```python
from build123d import *

# Parameters (mm, degrees)
SKETCH1_W                 = 105
SKETCH1_H                 = 65
BOSS_EXTRUDE1_DEPTH       = 40
FILLET1_R                 = 5
CUT_EXTRUDE1_DEPTH        = 38
SKETCH4_R                 = 2.5
SKETCH4_R_2               = 1
BOSS_EXTRUDE2_DEPTH       = 30
MIRROR2_COPY_1_SKETCH_R   = 2.5
MIRROR2_COPY_1_SKETCH_R_2 = 1
MIRROR2_COPY_1_DEPTH      = 30
CUT_EXTRUDE2_REACH        = 67
SKETCH7_R                 = 1.5
CUT_EXTRUDE3_REACH        = 4
SKETCH9_R                 = 2
CUT_EXTRUDE4_REACH        = 67
SKETCH12_R                = 3
FILLET2_R                 = 1
CUT_EXTRUDE5_REACH        = 67
SKETCH13_R                = 1.75


with BuildPart() as part:
    # Sketch1 → Boss-Extrude1 (new body)
    with BuildSketch(Plane(origin=(0, 0, 0), x_dir=(1, 0, 0), z_dir=(0, 1, 0))):
        with Locations((52.5, 32.5)):
            Rectangle(SKETCH1_W, SKETCH1_H)
    extrude(amount=BOSS_EXTRUDE1_DEPTH)

    # Fillet1
    fillet1_edges = [part.edges().sort_by_distance(p)[0] for p in [
        (0, 20, 0),
        (0, 20, -65),
        (105, 20, -65),
        (105, 20, 0),
    ]]
    fillet(fillet1_edges, radius=FILLET1_R)

    # Sketch3 → Cut-Extrude1 (cut)
    with BuildSketch(Plane(origin=(0, 40, 0), x_dir=(1, 0, 0), z_dir=(0, 1, 0))):
        with BuildLine():
            Line((100, 63), (5, 63))
            ThreePointArc((5, 63), (2.878679656, 62.121320344), (2, 60))
            Line((2, 60), (2, 5))
            ThreePointArc((2, 5), (2.878679656, 2.878679656), (5, 2))
            Line((5, 2), (100, 2))
            ThreePointArc((100, 2), (102.121320344, 2.878679656), (103, 5))
            Line((103, 5), (103, 60))
            ThreePointArc((103, 60), (102.121320344, 62.121320344), (100, 63))
        make_face()
    extrude(amount=-CUT_EXTRUDE1_DEPTH, mode=Mode.SUBTRACT)

    # Sketch4 → Boss-Extrude2 (add)
    with BuildSketch(Plane(origin=(0, 2, 0), x_dir=(1, 0, 0), z_dir=(0, 1, 0))):
        with Locations((99, 6)):
            Circle(SKETCH4_R)
        with Locations((99, 6)):
            Circle(SKETCH4_R_2, mode=Mode.SUBTRACT)
    boss_extrude2 = extrude(amount=BOSS_EXTRUDE2_DEPTH)

    # Mirror1: Boss-Extrude2 across plane
    add(boss_extrude2.mirror(Plane(origin=(0, 0, -32.5), x_dir=(1, 0, 0), z_dir=(0, 0, -1))))

    # Mirror2: Boss-Extrude2 across plane
    add(boss_extrude2.mirror(Plane.ZY.offset(-52.5)))

    # Mirror2 copy 1 sketch → Mirror2 copy 1 (add)
    with BuildSketch(Plane(origin=(105, 2, -65), x_dir=(-1, 0, 0), z_dir=(0, 1, 0))):
        with Locations((99, 6)):
            Circle(MIRROR2_COPY_1_SKETCH_R)
        with Locations((99, 6)):
            Circle(MIRROR2_COPY_1_SKETCH_R_2, mode=Mode.SUBTRACT)
    extrude(amount=MIRROR2_COPY_1_DEPTH)

    # Sketch7 → Cut-Extrude2 (cut, up to next)
    with BuildSketch(Plane.XY, mode=Mode.PRIVATE) as cut_extrude2_sk1:
        with Locations((89.576612985, 14.483747467)):
            Circle(SKETCH7_R)
    cut_extrude2_tool1 = extrude(cut_extrude2_sk1.sketch, amount=-CUT_EXTRUDE2_REACH, mode=Mode.PRIVATE) & part.part
    add(cut_extrude2_tool1.solids().sort_by_distance((89.576613, 14.483747, 0))[0], mode=Mode.SUBTRACT)
    # Sketch7 → Cut-Extrude2 (cut, up to next)
    with BuildSketch(Plane.XY, mode=Mode.PRIVATE) as cut_extrude2_sk2:
        with Locations((49.376612985, 14.483747467)):
            Circle(SKETCH7_R)
    cut_extrude2_tool2 = extrude(cut_extrude2_sk2.sketch, amount=-CUT_EXTRUDE2_REACH, mode=Mode.PRIVATE) & part.part
    add(cut_extrude2_tool2.solids().sort_by_distance((49.376613, 14.483747, 0))[0], mode=Mode.SUBTRACT)
    # Sketch7 → Cut-Extrude2 (cut, up to next)
    with BuildSketch(Plane.XY, mode=Mode.PRIVATE) as cut_extrude2_sk3:
        with BuildLine():
            Line((83.683719766, 19.28006781), (78.597933329, 24.365854248))
            ThreePointArc((78.597933329, 24.365854248), (78.27350998, 24.582626999), (77.890826547, 24.658747467))
            Line((77.890826547, 24.658747467), (61.062399423, 24.658747467))
            ThreePointArc((61.062399423, 24.658747467), (60.67971599, 24.582626999), (60.355292641, 24.365854248))
            Line((60.355292641, 24.365854248), (55.269506204, 19.28006781))
            ThreePointArc((55.269506204, 19.28006781), (55.052733452, 18.955644461), (54.976612985, 18.572961029))
            Line((54.976612985, 18.572961029), (54.976612985, 7.808747467))
            ThreePointArc((54.976612985, 7.808747467), (56.001739251, 5.333873733), (58.476612985, 4.308747467))
            Line((58.476612985, 4.308747467), (80.476612985, 4.308747467))
            ThreePointArc((80.476612985, 4.308747467), (82.951486719, 5.333873733), (83.976612985, 7.808747467))
            Line((83.976612985, 7.808747467), (83.976612985, 18.572961029))
            ThreePointArc((83.976612985, 18.572961029), (83.900492517, 18.955644461), (83.683719766, 19.28006781))
        make_face()
    cut_extrude2_tool3 = extrude(cut_extrude2_sk3.sketch, amount=-CUT_EXTRUDE2_REACH, mode=Mode.PRIVATE) & part.part
    add(cut_extrude2_tool3.solids().sort_by_distance((69.476613, 14.089774, 0))[0], mode=Mode.SUBTRACT)

    # Sketch9 → Cut-Extrude3 (cut, up to next)
    with BuildSketch(Plane(origin=(0, 2, 0), x_dir=(1, 0, 0), z_dir=(0, 1, 0)), mode=Mode.PRIVATE) as cut_extrude3_sk1:
        with Locations((93, 32.5)):
            Circle(SKETCH9_R)
    cut_extrude3_tool1 = extrude(cut_extrude3_sk1.sketch, amount=-CUT_EXTRUDE3_REACH, mode=Mode.PRIVATE) & part.part
    add(cut_extrude3_tool1.solids().sort_by_distance((93, 2, -32.5))[0], mode=Mode.SUBTRACT)
    # Sketch9 → Cut-Extrude3 (cut, up to next)
    with BuildSketch(Plane(origin=(0, 2, 0), x_dir=(1, 0, 0), z_dir=(0, 1, 0)), mode=Mode.PRIVATE) as cut_extrude3_sk2:
        with Locations((12, 32.5)):
            Circle(SKETCH9_R)
    cut_extrude3_tool2 = extrude(cut_extrude3_sk2.sketch, amount=-CUT_EXTRUDE3_REACH, mode=Mode.PRIVATE) & part.part
    add(cut_extrude3_tool2.solids().sort_by_distance((12, 2, -32.5))[0], mode=Mode.SUBTRACT)

    # Sketch12 → Cut-Extrude4 (cut, up to next)
    with BuildSketch(Plane.XY, mode=Mode.PRIVATE) as cut_extrude4_sk1:
        with Locations((25, 30)):
            Circle(SKETCH12_R)
    cut_extrude4_tool1 = extrude(cut_extrude4_sk1.sketch, amount=-CUT_EXTRUDE4_REACH, mode=Mode.PRIVATE) & part.part
    add(cut_extrude4_tool1.solids().sort_by_distance((25, 30, 0))[0], mode=Mode.SUBTRACT)

    # Fillet2
    fillet2_edges = [part.edges().sort_by_distance(p)[0] for p in [
        (22, 30, 0),
    ]]
    fillet(fillet2_edges, radius=FILLET2_R)

    # Sketch13 → Cut-Extrude5 (cut, up to next)
    with BuildSketch(Plane(origin=(0, 0, -65), x_dir=(-1, 0, 0), z_dir=(0, 0, -1)), mode=Mode.PRIVATE) as cut_extrude5_sk1:
        with Locations((-25, 30)):
            Circle(SKETCH13_R)
    cut_extrude5_tool1 = extrude(cut_extrude5_sk1.sketch, amount=-CUT_EXTRUDE5_REACH, mode=Mode.PRIVATE) & part.part
    add(cut_extrude5_tool1.solids().sort_by_distance((25, 30, -65))[0], mode=Mode.SUBTRACT)


solid = part.part
```
Can you work these out from the model? Positions are in its coordinate system, mm. A direction names the side the tool comes from. Round coordinates to 2 decimals unless told otherwise and drop trailing zeros. Loops run counter-clockwise (first coordinate to the right, second up) from the corner with the lowest first, then second, coordinate; pieces in that order, holes last. Notation, with made-up numbers: (58.25, 39.5) -> (71.25, 39.5) arc R25 cw to (71.25, 70.5) -> close; hole circle Ø11 at (-18, 32.25). An arc over 180 degrees is marked (long way). One line per item, written item: value. Start each with the question number.
1. For pin 1 (1.6 mm diameter, centred on x = 99, z = -59.5, fed in from +Y); pin 2 (1.6 mm diameter, centred on y = 13.5, z = -1, fed in from -X); pin 3 (5 mm diameter, centred on x = 12, z = -32.5, fed in from +Y), each with a flat end and sliding along its axis, tell me the tip position at first contact or that it passes through.
2. If we section it at D-D, the plane x = 25.5: Give the number of separate pieces and of enclosed holes in the cut face, then the cut area to 3 significant figures.
3. If we section it at A-A, the plane z = -32.5: Write out the boundary of the cut face in (x, y).
4. If I drill on probe 1 along Z at (x, y) = (6, 23); probe 2 along X at (y, z) = (33.5, -50); probe 3 along Z at (x, y) = (19, 20), over which ranges is the centre line in solid material (lowest first)?
5. If we section it at B-B, the plane x = 93: Write out the boundary of the cut face in (y, z).
6. If we mould it in two halves opening along X, with no side actions, what happens to faces 1 (the flat face through (83.977, 13, -1)), 2 (the cylindrical face through (103, 20, -1)), 3 (the cylindrical face through (1, 20, -63))? For each: pulls with the +X half, pulls with the -X half, needs draft (parallel to the pull), parting line crosses it, or undercut.
7. If we section it at C-C, the plane z = -46.5: Write out the boundary of the cut face in (x, y), then the cut area to 3 significant figures.
8. For faces 4 (the cylindrical face through (98, 17, -59)), 5 (the cylindrical face through (11.566, 1.014, -30.548)), 6 (the flat face through (54.977, 13, -1)), which set-ups out of +Z, -Z, +X, -X, +Y, -Y let a thin tool reach every point of the face, with its end or its side?
Calculated:
1. pin 1: stops at y = 32
1. pin 2: stops at x = 1.16
1. pin 3: stops at y = 2
2. separate pieces: 3
2. enclosed holes: 0
2. area: 263 mm²
3. outline: (0, 0) -> (10, 0) -> (10, 2) -> (2, 2) -> (2, 40) -> (0, 40) -> close; (14, 0) -> (91, 0) -> (91, 2) -> (14, 2) -> close; (95, 0) -> (105, 0) -> (105, 40) -> (103, 40) -> (103, 2) -> (95, 2) -> close
4. probe 1: z = -65 to -63, -61.5 to -60, -58 to -56.5, -8.5 to -7, -5 to -3.5, -2 to 0
4. probe 2: x = 0 to 2, 103 to 105
4. probe 3: z = -65 to -63, -2 to 0
5. outline: (0, -65) -> (40, -65) -> (40, -63) -> (2, -63) -> (2, -34.5) -> (0, -34.5) -> close; (0, -30.5) -> (2, -30.5) -> (2, -2) -> (40, -2) -> (40, 0) -> (0, 0) -> close
6. face 1: undercut
6. face 2: pulls with the +X half
6. face 3: pulls with the -X half
7. outline: (0, 0) -> (105, 0) -> (105, 40) -> (103, 40) -> (103, 2) -> (2, 2) -> (2, 40) -> (0, 40) -> close
7. area: 362 mm²
8. face 4: +Y
8. face 5: +Y, -Y
8. face 6: +Z
